```python
from build123d import *

# Parameters (mm, degrees)
SKETCH1_W           = 30
SKETCH1_H           = 25
BOSS_EXTRUDE1_DEPTH = 25
CUT_EXTRUDE1_DEPTH  = 26
CUT_EXTRUDE2_DEPTH  = 10


with BuildPart() as part:
    # Sketch1 → Boss-Extrude1 (new body)
    with BuildSketch(Plane.XY):
        Rectangle(SKETCH1_W, SKETCH1_H)
    extrude(amount=BOSS_EXTRUDE1_DEPTH)

    # Sketch3 → Cut-Extrude1 (cut, through all)
    with BuildSketch(Plane.XY.offset(25)):
        Polygon((15, 12.5), (-15, 2.5), (-15, 12.5), align=None)
    extrude(amount=-CUT_EXTRUDE1_DEPTH, mode=Mode.SUBTRACT)

    # Sketch4 → Cut-Extrude2 (cut)
    with BuildSketch(Plane(origin=(0, 0, 0), x_dir=(-1, 0, 0), z_dir=(0, 0, -1))):
        Polygon((-15, 12.5), (-15, 7.5), (15, -7.5), (15, 2.5), align=None)
    extrude(amount=-CUT_EXTRUDE2_DEPTH, mode=Mode.SUBTRACT)


solid = part.part
```
Input: part model. Units: mm. Frame: model coordinates. A direction names the side the tool comes from. Round coordinates to 2 decimals unless told otherwise and drop trailing zeros. Order: outer loops, then holes, each group sorted by start corner. A loop starts at its lowest first (then second) coordinate and runs counter-clockwise, first axis right, second up. Notation, with made-up numbers: (-36, 2.5) - (-8, 2.5) arc R24 ccw to (-8, 32.5) - close; hole circle Ø4 at (11.25, -27.75). An arc over 180 degrees is marked (long way). One line per question, with ' | ' between items. Start each with the question number.
1) Ray query, probe 1 along Z at (x, y) = (-5, 3); probe 2 along X at (y, z) = (-3, 2.5); probe 3 along Y at (x, z) = (-7.5, 2). Return the intervals inside material, ascending.
2) Cut plane D-D, the plane y = 10.25. Return the cut outline in (x, z).
3) Cut plane C-C, the plane z = 6. Return the cut outline in (x, y).
4) Contact query for flat-ended pins moving along their axis: P1, Ø5, axis at x = 10, z = 12.5, coming from the +Y side; P2, Ø3, axis at y = -3, z = 7.5, coming from the -X side; P3, Ø4, axis at x = -4, z = 3, coming from the +Y side. Output: stop coordinate, or through.
5) Cut plane B-B, the plane y = 0.5. Return the cut outline in (x, z).
6) Cut plane A-A, the plane x = 7.5. Return the cut outline in (y, z).
7) Set-up query: faces 1 (the flat face through (0.21, 7.57, 17.6)), 2 (the flat face through (0, 0, 5)). Return all of +Z, -Z, +X, -X, +Y, -Y with unobstructed straight access to the full face (end or side cutting, diameter ignored); none if empty.
Worked out:
1) probe 1: z = 10 to 25 | probe 2: x = -6 to 15 | probe 3: y = -12.5 to -3.75
2) outline: (8.25, 10) - (15, 10) - (15, 25) - (8.25, 25) - close
3) outline: (-15, -12.5) - (15, -12.5) - (15, 7.5) - (-15, -7.5) - close
4) P1: stops at y = 11.67 | P2: stops at x = -9 | P3: stops at y = -1
5) outline: (-15, 10) - (1, 10) - (1, 0) - (15, 0) - (15, 25) - (-15, 25) - close
6) outline: (-12.5, 0) - (3.75, 0) - (3.75, 10) - (10, 10) - (10, 25) - (-12.5, 25) - close
7) face 1: +Z, -Z, -X, +Y | face 2: -Z, -X, +Y
